from build123d import *

# Parameters (mm, degrees)
SKETCH1_W           = 55.8
SKETCH1_H           = 15.8
BOSS_EXTRUDE1_DEPTH = 28.8
SKETCH2_R           = 7.62
CUT_EXTRUDE1_DEPTH  = 12.7
SKETCH4_R           = 2.778125
SKETCH4_R_2         = 1.8415
CUT_EXTRUDE2_DEPTH  = 12.7
CUT_EXTRUDE6_DEPTH  = 1.905
SKETCH8_W           = 53.36
SKETCH8_H           = 13.36
SKETCH8_R           = 3.26
CUT_EXTRUDE8_DEPTH  = 2.23
SKETCH11_R          = 2.405
BOSS_EXTRUDE3_DEPTH = 1.9


with BuildPart() as part:
    # Sketch1 → Boss-Extrude1 (new body)
    with BuildSketch(Plane(origin=(0, 0, 0), x_dir=(1, 0, 0), z_dir=(0, 1, 0))):
        with Locations((-11.199948696, 8.193463303)):
            Rectangle(SKETCH1_W, SKETCH1_H)
    extrude(amount=BOSS_EXTRUDE1_DEPTH)

    # Sketch2 → Cut-Extrude1 (cut)
    with BuildSketch(Plane.XY.offset(-0.293463303)):
        with Locations((0.800051304, 13.4)):
            Circle(SKETCH2_R)
        with BuildLine():
            Line((-11.899948696, 8.6375), (-24.599948696, 8.6375))
            ThreePointArc((-24.599948696, 8.6375), (-29.362448696, 13.4), (-24.599948696, 18.1625))
            Line((-24.599948696, 18.1625), (-11.899948696, 18.1625))
            ThreePointArc((-11.899948696, 18.1625), (-7.137448696, 13.4), (-11.899948696, 8.6375))
        make_face()
    extrude(amount=-CUT_EXTRUDE1_DEPTH, mode=Mode.SUBTRACT)

    # Sketch4 → Cut-Extrude2 (cut)
    with BuildSketch(Plane(origin=(0, 0, -16.093463303), x_dir=(-1, 0, 0), z_dir=(0, 0, -1))):
        with Locations((-0.800051304, 13.4)):
            Circle(SKETCH4_R)
        with Locations((11.899948696, 13.4)):
            Circle(SKETCH4_R_2)
        with Locations((24.599948696, 13.4)):
            Circle(SKETCH4_R_2)
    extrude(amount=-CUT_EXTRUDE2_DEPTH, mode=Mode.SUBTRACT)

    # Sketch5 → Cut-Extrude6 (cut)
    with BuildSketch(Plane(origin=(0, 0, -16.093463303), x_dir=(-1, 0, 0), z_dir=(0, 0, -1))):
        with BuildLine():
            Line((24.599948696, 18.1625), (11.899948696, 18.1625))
            ThreePointArc((11.899948696, 18.1625), (7.137448696, 13.4), (11.899948696, 8.6375))
            Line((11.899948696, 8.6375), (24.599948696, 8.6375))
            ThreePointArc((24.599948696, 8.6375), (29.362448696, 13.4), (24.599948696, 18.1625))
        make_face()
    extrude(amount=-CUT_EXTRUDE6_DEPTH, mode=Mode.SUBTRACT)

    # Sketch8 → Cut-Extrude8 (cut)
    with BuildSketch(Plane(origin=(0, 28.8, 0), x_dir=(1, 0, 0), z_dir=(0, 1, 0))):
        with Locations((-11.199948696, 8.193463303)):
            Rectangle(SKETCH8_W, SKETCH8_H)
        with Locations((-31.199948696, 8.193463303)):
            Circle(SKETCH8_R, mode=Mode.SUBTRACT)
        with Locations((-23.199948696, 8.193463303)):
            Circle(SKETCH8_R, mode=Mode.SUBTRACT)
        with Locations((-15.199948696, 8.193463303)):
            Circle(SKETCH8_R, mode=Mode.SUBTRACT)
        with Locations((-7.199948696, 8.193463303)):
            Circle(SKETCH8_R, mode=Mode.SUBTRACT)
        with Locations((0.800051304, 8.193463303)):
            Circle(SKETCH8_R, mode=Mode.SUBTRACT)
        with Locations((8.800051304, 8.193463303)):
            Circle(SKETCH8_R, mode=Mode.SUBTRACT)
    extrude(amount=-CUT_EXTRUDE8_DEPTH, mode=Mode.SUBTRACT)

    # Sketch11 → Boss-Extrude3 (add)
    with BuildSketch(Plane.XZ):
        with Locations((-35.199948696, -4.193463303)):
            Circle(SKETCH11_R)
        with Locations((-35.199948696, -12.193463303)):
            Circle(SKETCH11_R)
        with Locations((-27.199948696, -4.193463303)):
            Circle(SKETCH11_R)
        with Locations((-27.199948696, -12.193463303)):
            Circle(SKETCH11_R)
        with Locations((-19.199948696, -4.193463303)):
            Circle(SKETCH11_R)
        with Locations((-19.199948696, -12.193463303)):
            Circle(SKETCH11_R)
        with Locations((-11.199948696, -4.193463303)):
            Circle(SKETCH11_R)
        with Locations((-11.199948696, -12.193463303)):
            Circle(SKETCH11_R)
        with Locations((-3.199948696, -4.193463303)):
            Circle(SKETCH11_R)
        with Locations((-3.199948696, -12.193463303)):
            Circle(SKETCH11_R)
        with Locations((4.800051304, -4.193463303)):
            Circle(SKETCH11_R)
        with Locations((4.800051304, -12.193463303)):
            Circle(SKETCH11_R)
        with Locations((12.800051304, -4.193463303)):
            Circle(SKETCH11_R)
        with Locations((12.800051304, -12.193463303)):
            Circle(SKETCH11_R)
    extrude(amount=BOSS_EXTRUDE3_DEPTH)


solid = part.part
Could you check a few things on this model? Use its own coordinates, in mm. A direction names the side the tool comes from. Give positions to 0.01 mm unless a question says otherwise; leave off trailing zeros. Write each loop counter-clockwise with the first axis right and the second up, starting at its lowest first coordinate (ties: lowest second). Pieces come first, ordered by that corner, then holes. Notation, with made-up numbers: (25, -25) -> (50, -25) arc R10 cw to (50, -10) -> close; hole circle Ø8 at (-8.75, 0.25). An arc over 180 degrees is marked (long way). Answer as a JSON object with one key per item and string values.
Q1. Please list where these lines run through material, in increasing order: L1, parallel to Y at x = -20, z = -8.25; L2, parallel to Y at x = -16, z = -4; L3, parallel to X at y = 12.5, z = -14.5.
Taken from the geometry:
{"L1": "y = 0 to 8.64, 18.16 to 28.8", "L2": "y = 0 to 8.64, 18.16 to 26.57", "L3": "x = -39.1 to -29.28, -7.22 to -1.83, 3.43 to 16.7"}
Q2. Suppose I cut it at A-A on y = 13.4. Write out the boundary of the cut face in (x, z).
Taken from the geometry:
{"outline": "(-39.1, -16.09) -> (-29.36, -16.09) -> (-29.36, -14.19) -> (-26.44, -14.19) -> (-26.44, -12.99) -> (-29.36, -12.99) -> (-29.36, -0.29) -> (-39.1, -0.29) -> close; (-22.76, -14.19) -> (-13.74, -14.19) -> (-13.74, -12.99) -> (-22.76, -12.99) -> close; (-10.06, -14.19) -> (-7.14, -14.19) -> (-7.14, -16.09) -> (-1.98, -16.09) -> (-1.98, -12.99) -> (-6.82, -12.99) -> (-6.82, -0.29) -> (-7.14, -0.29) -> (-7.14, -12.99) -> (-10.06, -12.99) -> close; (3.58, -16.09) -> (16.7, -16.09) -> (16.7, -0.29) -> (8.42, -0.29) -> (8.42, -12.99) -> (3.58, -12.99) -> close"}
Q3. Which directions (+Z, -Z, +X, -X, +Y, -Y) give clear straight access to the entire face, cutting with the end or side of a thin tool? Please do faces 4 (the flat face through (-18, 18.162, -15)), 5 (the flat face through (-18, 13, -12.993)), 6 (the flat face through (-12, 0, -8)).
Taken from the geometry:
{"face 4": "-Z", "face 5": "+Z", "face 6": "-Y"}
Q4. Will these pins go through, and if not, where does the flat tip stop? pin 1 Ø0.6 at (x, z) = (-18, -15.5) entering from -Y; pin 2 Ø4 at (x, y) = (-24.6, 13.4) entering from +Z.
Taken from the geometry:
{"pin 1": "stops at y = 0", "pin 2": "stops at z = -12.99"}
Q5. Suppose I cut it at C-C on x = 5. Write out the boundary of the cut face in (y, z), then the cut area to 3 significant figures.
Taken from the geometry:
{"outline": "(-1.9, -14.59) -> (0, -14.59) -> (0, -16.09) -> (28.8, -16.09) -> (28.8, -14.87) -> (26.57, -14.87) -> (26.57, -1.51) -> (28.8, -1.51) -> (28.8, -0.29) -> (19.76, -0.29) -> (19.76, -12.99) -> (7.04, -12.99) -> (7.04, -0.29) -> (0, -0.29) -> (0, -1.8) -> (-1.9, -1.8) -> (-1.9, -6.59) -> (0, -6.59) -> (0, -9.8) -> (-1.9, -9.8) -> close", "area": "282 mm²"}
Q6. We'd pull the mould along X, two halves only. Please class faces 1 (the flat face through (-39.1, 14, -8)), 2 (the flat face through (-5, 14, -16.093)), 3 (the flat face through (-18, 18.162, -7)): released by +X, released by -X, zero draft, split by the parting line, or undercut.
Taken from the geometry:
{"face 1": "released by -X", "face 2": "zero draft", "face 3": "undercut"}
Q7. Suppose I cut it at D-D on y = 17.5. Write out the boundary of the cut face in (x, z).
Taken from the geometry:
{"outline": "(-39.1, -16.09) -> (-27.02, -16.09) -> (-27.02, -14.19) -> (-9.48, -14.19) -> (-9.48, -16.09) -> (16.7, -16.09) -> (16.7, -0.29) -> (7.22, -0.29) -> (7.22, -12.99) -> (-5.62, -12.99) -> (-5.62, -0.29) -> (-9.48, -0.29) -> (-9.48, -12.99) -> (-27.02, -12.99) -> (-27.02, -0.29) -> (-39.1, -0.29) -> close"}
Q8. Suppose I cut it at B-B on x = -24. Write out the boundary of the cut face in (y, z).
Taken from the geometry:
{"outline": "(0, -16.09) -> (8.64, -16.09) -> (8.64, -14.19) -> (11.66, -14.19) -> (11.66, -12.99) -> (8.64, -12.99) -> (8.64, -0.29) -> (0, -0.29) -> close; (15.14, -14.19) -> (18.16, -14.19) -> (18.16, -16.09) -> (28.8, -16.09) -> (28.8, -14.87) -> (26.57, -14.87) -> (26.57, -11.35) -> (28.8, -11.35) -> (28.8, -5.03) -> (26.57, -5.03) -> (26.57, -1.51) -> (28.8, -1.51) -> (28.8, -0.29) -> (18.16, -0.29) -> (18.16, -12.99) -> (15.14, -12.99) -> close"}
